Source: CAD feature listing. Evaluate the final solid. Frame: model axes, mm. Round coordinates to 2 decimals unless told otherwise and drop trailing zeros. Write each loop counter-clockwise with the first axis right and the second up, starting at its lowest first coordinate (ties: lowest second). Pieces come first, ordered by that corner, then holes. Notation, with made-up numbers: (-30, 55) -> (3, 55) arc R21 ccw to (3, 75) -> close; hole circle Ø3 at (89, -0.5). An arc over 180 degrees is marked (long way). Return JSON: item names as keys, results as strings. Group by question number.
from build123d import *

# Parameters (mm, degrees)
SKETCH1_R           = 3.5
BASEHEAD_DEPTH      = 4
SKETCH2_R           = 2
BASEBODY_DEPTH      = 20
HEXAGONSOCKET_DEPTH = 2
TOPFILLET_R         = 0.5
CHAMFER1_SIZE       = 0.2
LPATTERN10_COUNT    = 44
LPATTERN10_PITCH    = 0.4548


with BuildPart() as part:
    # Sketch1 → BaseHead (new body)
    with BuildSketch(Plane(origin=(0, 0, 0), x_dir=(0, 0, -1), z_dir=(1, 0, 0))):
        Circle(SKETCH1_R)
    extrude(amount=BASEHEAD_DEPTH)

    # Sketch2 → BaseBody (add)
    with BuildSketch(Plane(origin=(4, 0, 0), x_dir=(0, 0, -1), z_dir=(1, 0, 0))):
        Circle(SKETCH2_R)
    extrude(amount=BASEBODY_DEPTH)

    # Sketch3 → HexagonSocket (cut)
    with BuildSketch(Plane(origin=(0, 0, 0), x_dir=(0, 0, -1), z_dir=(1, 0, 0))):
        Polygon((1.732050808, 0), (0.866025404, 1.5), (-0.866025404, 1.5), (-1.732050808, 0), (-0.866025404, -1.5), (0.866025404, -1.5), align=None)
    extrude(amount=HEXAGONSOCKET_DEPTH, mode=Mode.SUBTRACT)

    # Sketch4 → Cut-Revolve1 (revolve, cut)
    with BuildSketch(Plane(origin=(-4.19613823, 0.75, 0), x_dir=(-1, 0, 0), z_dir=(0, 0, 1))):
        Polygon((-6.19613823, 2.25), (-7.062163633, 0.75), (-6.19613823, 0.75), align=None)
    revolve(axis=Axis((0.838992387, 0, 0), (-1, 0, 0)), mode=Mode.SUBTRACT)

    # TopFillet
    topfillet_edges = [part.edges().sort_by_distance(p)[0] for p in [
        (0, 0, 3.5),
    ]]
    fillet(topfillet_edges, radius=TOPFILLET_R)

    # Chamfer1
    chamfer1_edges = [part.edges().sort_by_distance(p)[0] for p in [
        (24, 0, 2),
    ]]
    chamfer(chamfer1_edges, length=CHAMFER1_SIZE)

    # Sketch5 → Cut-Revolve10 (revolve, cut)
    with BuildSketch(Plane.XY):
        Polygon((23.8, 1.671776372), (23.9895, 2), (23.9895, 2.379), (23.6105, 2.379), (23.6105, 2), align=None)
    cut_revolve10 = revolve(axis=Axis((0, 0, 0), (1, 0, 0)), mode=Mode.SUBTRACT)

    # LPattern10: Cut-Revolve10 ×44
    with Locations(*[(-i * LPATTERN10_PITCH, 0, 0) for i in range(1, LPATTERN10_COUNT)]):
        add(cut_revolve10, mode=Mode.SUBTRACT)


solid = part.part
Item 1: Material intervals for probe 1 along X at (y, z) = (0, -2.5); probe 2 along X at (y, z) = (0, -1.5); probe 3 along Z at (x, y) = (15.5, 1), sorted ascending.
Item 2: Cut plane A-A on x = 3.5. Output: boundary loops of the cut face in (y, z), and give its area (3 significant figures).
Item 3: First-contact query: pin 1 Ø1.5 at (x, z) = (19.5, -0.5) entering from +Y; pin 2 Ø3 at (x, y) = (11.5, -2) entering from +Z. Flat tips, straight axial feed; report the tip coordinate or a pass-through.
Here are the results:
{
 "1": {"probe 1": "x = 0 to 4", "probe 2": "x = 2 to 24", "probe 3": "z = -1.58 to 1.58"},
 "2": {"outline": "circle Ø7 at (0, 0)", "area": "38.5 mm^2"},
 "3": {"pin 1": "stops at y = 2", "pin 2": "stops at z = 1.93"}
}
